Input: part model. Units: mm. Frame: model coordinates. Face numbers are marked on the shaded views. Round coordinates to 2 decimals unless told otherwise and drop trailing zeros. Order: outer loops, then holes, each group sorted by start corner. A loop starts at its lowest first (then second) coordinate and runs counter-clockwise, first axis right, second up. Notation, with made-up numbers: (-8.75, 7.5) -> (16.25, 7.5) arc R13 ccw to (16.25, 27.5) -> close; hole circle Ø5 at (-12, 38). An arc over 180 degrees is marked (long way). Use a Markdown table: item, result.
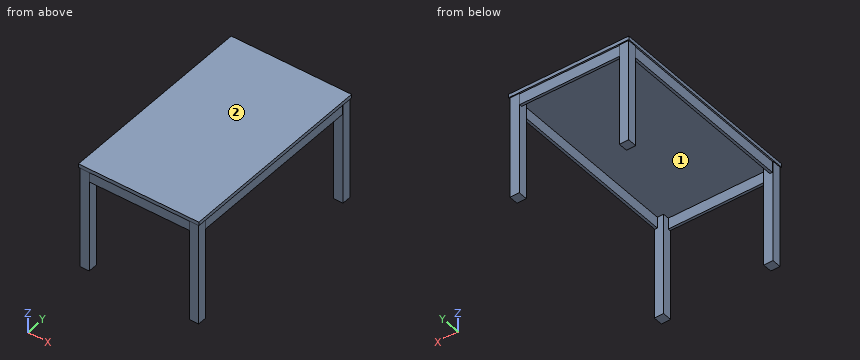
from build123d import *

# Parameters (mm, degrees)
F0_W     = 840
F0_H     = 1400
F1_DEPTH = 25
F3_DEPTH = 715
F2_W     = 18
F2_H     = 1258
F2_W_2   = 698
F2_H_2   = 18
F4_DEPTH = 78


with BuildPart() as f1:
    # F0 (on Top) → F1 (new body)
    with BuildSketch(Plane.XY):
        Rectangle(F0_W, F0_H)
    extrude(amount=F1_DEPTH)

    # F2 (on face) → F3 (join)
    with BuildSketch(Plane(origin=(0, 0, 0), x_dir=(1, 0, 0), z_dir=(0, 0, -1))):
        Polygon((349, 672), (349, 629), (392, 629), (410, 629), (414, 629), (414, 694), (349, 694), (349, 690), align=None)
        Polygon((410, -629), (392, -629), (349, -629), (349, -672), (349, -690), (349, -694), (414, -694), (414, -629), align=None)
        Polygon((-349, -690), (-349, -672), (-349, -629), (-392, -629), (-410, -629), (-414, -629), (-414, -694), (-349, -694), align=None)
        Polygon((-349, 629), (-349, 672), (-349, 690), (-349, 694), (-414, 694), (-414, 629), (-410, 629), (-392, 629), align=None)
    extrude(amount=F3_DEPTH)

    # F2 (on face) → F4 (join)
    with BuildSketch(Plane(origin=(0, 0, 0), x_dir=(1, 0, 0), z_dir=(0, 0, -1))):
        with Locations((401, 0)):
            Rectangle(F2_W, F2_H)
        with Locations((0, 681)):
            Rectangle(F2_W_2, F2_H_2)
        with Locations((-401, 0)):
            Rectangle(F2_W, F2_H)
        with Locations((0, -681)):
            Rectangle(F2_W_2, F2_H_2)
    extrude(amount=F4_DEPTH)


solid = f1.part
1) Cut plane C-C on x = -291. Return loops of the section in (y, z).
Answer key:
| item | result |
|---|---|
| outline | (-700, 0) -> (-690, 0) -> (-690, -78) -> (-672, -78) -> (-672, 0) -> (672, 0) -> (672, -78) -> (690, -78) -> (690, 0) -> (700, 0) -> (700, 25) -> (-700, 25) -> close |
2) Contact query for flat-ended pins moving along their axis: P1, Ø5.5, axis at x = -135.5, y = 682.5, coming from the -Z side; P2, Ø23.5, axis at x = -87.5, z = -55.5, coming from the +Y side; P3, Ø19.5, axis at y = 653, z = -375, coming from the -X side. Output: stop coordinate, or through.
Answer key:
| item | result |
|---|---|
| P1 | stops at z = -78 |
| P2 | stops at y = 690 |
| P3 | stops at x = -414 |
3) Cut plane B-B on y = -153.5. Return loops of the section in (x, z), and give its area (3 significant figures).
Answer key:
| item | result |
|---|---|
| outline | (-420, 0) -> (-410, 0) -> (-410, -78) -> (-392, -78) -> (-392, 0) -> (392, 0) -> (392, -78) -> (410, -78) -> (410, 0) -> (420, 0) -> (420, 25) -> (-420, 25) -> close |
| area | 23,800 mm^2 |
4) Cut plane A-A on z = -518. Return loops of the section in (x, y).
Answer key:
| item | result |
|---|---|
| outline | (-414, -694) -> (-349, -694) -> (-349, -629) -> (-414, -629) -> close; (-414, 629) -> (-349, 629) -> (-349, 694) -> (-414, 694) -> close; (349, -694) -> (414, -694) -> (414, -629) -> (349, -629) -> close; (349, 629) -> (414, 629) -> (414, 694) -> (349, 694) -> close |
5) Ray query, probe 1 along Y at (x, z) = (-243, -27); probe 2 along X at (y, z) = (390.5, -32.5); probe 3 along Z at (x, y) = (223, 534). Return the intervals inside material, ascending.
Answer key:
| item | result |
|---|---|
| probe 1 | y = -690 to -672, 672 to 690 |
| probe 2 | x = -410 to -392, 392 to 410 |
| probe 3 | z = 0 to 25 |
6) Draft query along X for the marked faces 1 and 2. Return one class per face: released by +X, released by -X, zero draft, split by the parting line, or undercut.
Answer key:
| item | result |
|---|---|
| face 1 | undercut |
| face 2 | zero draft |
